Build history of the part. All positions in model axes, mm. A direction names the side the tool comes from. Give positions to 0.01 mm unless a question says otherwise; leave off trailing zeros. Loops run counter-clockwise (first coordinate to the right, second up) from the corner with the lowest first, then second, coordinate; pieces in that order, holes last. Notation, with made-up numbers: M 45.25,42 L 80.25,42 A17 ccw 80.25,54 Z; hole C 21,19.5 d5. An arc over 180 degrees is marked long. Put each result on its own line as item: value.
```python
from build123d import *

# Parameters (mm, degrees)
BOSS_EXTRUDE1_DEPTH = 2.5
SKETCH2_R           = 1
CUT_EXTRUDE1_DEPTH  = 5
SKETCH3_R           = 1
CUT_EXTRUDE2_DEPTH  = 5
SKETCH4_R           = 1
BOSS_EXTRUDE2_DEPTH = 5
SKETCH6_W           = 2.5
SKETCH6_H           = 2.5
BOSS_EXTRUDE3_DEPTH = 25
SKETCH7_R           = 1
CUT_EXTRUDE3_DEPTH  = 5
SKETCH8_W           = 8
SKETCH8_H           = 2.5
CUT_EXTRUDE4_DEPTH  = 10
SKETCH9_R           = 1
CUT_EXTRUDE5_DEPTH  = 5
SKETCH10_R          = 1
BOSS_EXTRUDE4_DEPTH = 5
SKETCH11_W          = 2.5
SKETCH11_H          = 2.5
BOSS_EXTRUDE5_DEPTH = 1
SKETCH12_W          = 2.5
SKETCH12_H          = 2.5
BOSS_EXTRUDE6_DEPTH = 1
SKETCH13_W          = 2.5
SKETCH13_H          = 2.5
CUT_EXTRUDE6_DEPTH  = 1
CUT_EXTRUDE7_DEPTH  = 5


with BuildPart() as part:
    # Sketch1 → Boss-Extrude1 (new body)
    with BuildSketch(Plane.XY):
        Polygon((-13.3, 0), (0, 0), (3.830222216, 3.213938048), (5.465982834, 1.323359513), (0.909480399, -2.5), (-13.3, -2.5), align=None)
    extrude(amount=BOSS_EXTRUDE1_DEPTH)

    # Sketch2 → Cut-Extrude1 (cut)
    with BuildSketch(Plane(origin=(3.780724263, 3.271146765, 0), x_dir=(0, 0, -1), z_dir=(0.7562314141303861, 0.6543042474891605, 0))):
        with Locations(Location((-1.25, -1.325649749, 0), (0, 0, 90))):
            Circle(SKETCH2_R)
    extrude(amount=-CUT_EXTRUDE1_DEPTH, mode=Mode.SUBTRACT)

    # Sketch3 → Cut-Extrude2 (cut)
    with BuildSketch(Plane.ZY.offset(13.3)):
        with Locations((1.25, -1.25)):
            Circle(SKETCH3_R)
    extrude(amount=-CUT_EXTRUDE2_DEPTH, mode=Mode.SUBTRACT)

    # Sketch4 → Boss-Extrude2 (add)
    with BuildSketch(Plane.ZY.offset(13.3)):
        with Locations((1.25, -1.25)):
            Circle(SKETCH4_R)
    extrude(amount=-BOSS_EXTRUDE2_DEPTH)

    # Sketch6 → Boss-Extrude3 (add)
    with BuildSketch(Plane.ZY.offset(13.3)):
        with Locations((1.25, -1.25)):
            Rectangle(SKETCH6_W, SKETCH6_H)
    extrude(amount=BOSS_EXTRUDE3_DEPTH)

    # Sketch7 → Cut-Extrude3 (cut)
    with BuildSketch(Plane.ZY.offset(38.3)):
        with Locations((1.25, -1.25)):
            Circle(SKETCH7_R)
    extrude(amount=-CUT_EXTRUDE3_DEPTH, mode=Mode.SUBTRACT)

    # Sketch8 → Cut-Extrude4 (cut)
    with BuildSketch(Plane(origin=(0, 0, 0), x_dir=(-1, 0, 0), z_dir=(0, 0, -1))):
        with Locations((34.3, -1.25)):
            Rectangle(SKETCH8_W, SKETCH8_H)
    extrude(amount=-CUT_EXTRUDE4_DEPTH, mode=Mode.SUBTRACT)

    # Sketch9 → Cut-Extrude5 (cut)
    with BuildSketch(Plane.ZY.offset(30.3)):
        with Locations((1.25, -1.25)):
            Circle(SKETCH9_R)
    extrude(amount=-CUT_EXTRUDE5_DEPTH, mode=Mode.SUBTRACT)

    # Sketch10 → Boss-Extrude4 (add)
    with BuildSketch(Plane.ZY.offset(30.3)):
        with Locations((1.25, -1.25)):
            Circle(SKETCH10_R)
    extrude(amount=-BOSS_EXTRUDE4_DEPTH)

    # Sketch11 → Boss-Extrude5 (add)
    with BuildSketch(Plane.ZY.offset(30.3)):
        with Locations((1.25, -1.25)):
            Rectangle(SKETCH11_W, SKETCH11_H)
    extrude(amount=BOSS_EXTRUDE5_DEPTH)

    # Sketch12 → Boss-Extrude6 (add)
    with BuildSketch(Plane.ZY.offset(31.3)):
        with Locations((1.25, -1.25)):
            Rectangle(SKETCH12_W, SKETCH12_H)
    extrude(amount=BOSS_EXTRUDE6_DEPTH)

    # Sketch13 → Cut-Extrude6 (cut)
    with BuildSketch(Plane.ZY.offset(32.3)):
        with Locations((1.25, -1.25)):
            Rectangle(SKETCH13_W, SKETCH13_H)
    extrude(amount=-CUT_EXTRUDE6_DEPTH, mode=Mode.SUBTRACT)

    # Sketch14 → Cut-Extrude7 (cut)
    with BuildSketch(Plane.ZY.offset(31.3)):
        with BuildLine():
            ThreePointArc((2.25, -1.25), (1.25, -0.25), (0.25, -1.25))
            Line((0.25, -1.25), (2.25, -1.25))
        make_face()
        with BuildLine():
            Line((2.25, -1.25), (0.25, -1.25))
            ThreePointArc((0.25, -1.25), (1.25, -2.25), (2.25, -1.25))
        make_face()
    extrude(amount=-CUT_EXTRUDE7_DEPTH, mode=Mode.SUBTRACT)


solid = part.part
```
Q1. Tool access for faces 1 (the flat face through (-26.3, -1, 1)), 2 (the flat face through (0.876, -1.013, 1.264)), 3 (the flat face through (-15, -2.5, 1)): list every direction of +Z, -Z, +X, -X, +Y, -Y with a clear straight run to the whole face (end or side of a thin tool).
Here are the results:
face 1: -X
face 2: none
face 3: +Z, -Z, +X, -X, -Y
Q2. Slice it at B-B (x = -4). List the corners of the cut face in (y, z), and give its area (3 significant figures).
Here are the results:
outline: M -2.5,0 L 0,0 L 0,2.5 L -2.5,2.5 Z
area: 6.25 mm²
Q3. Probe line 1 (Y direction, x = -28.55, z = 1.25); line 2 (Z direction, x = -29.4, y = -1.25); line 3 (Y direction, x = -16.5, z = 1.65). List the from-to ranges inside material, lowest first. Write a range as from..to.
Here are the results:
line 1: -2.5..-2.25, -0.25..0
line 2: 0..0.25, 2.25..2.5
line 3: -2.5..0
Q4. Mould opens along Y. For faces 4 (the flat face through (-13, -1, 0)), 5 (the cylindrical face through (2.926, 0.492, 0.274)), 6 (the flat face through (-15, 0, 1)) say: pulls with the +Y half, pulls with the -Y half, needs draft (parallel to the pull), parting line crosses it, or undercut.
Here are the results:
face 4: needs draft
face 5: undercut
face 6: pulls with the +Y half
Q5. Slice it at A-A (z = 1.25). List the corners of the cut face in (x, y), and give its area (3 significant figures).
Here are the results:
outline: M -31.3,-2.5 L 0.91,-2.5 L 5.47,1.32 L 5.3,1.51 L 1.52,-1.76 L 0.21,-0.25 L 3.99,3.02 L 3.83,3.21 L 0,0 L -31.3,0 L -31.3,-0.25 L -26.3,-0.25 L -26.3,-2.25 L -31.3,-2.25 Z
area: 73.1 mm²
Q6. Drop flat-ended pins along their axis: pin 1 Ø3 at (x, y) = (-10, 1) entering from +Z; pin 2 Ø1.2 at (x, z) = (-9.5, 1) entering from +Y; pin 3 Ø1 at (y, z) = (-1, 1) entering from -X. Give the stop position or say it passes through.
Here are the results:
pin 1: z = 2.5
pin 2: y = 0
pin 3: x = -26.3
